Geometry: see drawing. Coordinates: mm, zero at the bounding-box minimum. Round coordinates to 2 decimals unless told otherwise and drop trailing zeros. Loops run counter-clockwise (first coordinate to the right, second up) from the corner with the lowest first, then second, coordinate; pieces in that order, holes last. Notation, with made-up numbers: (81, 79.5) - (136, 79.5) arc R14 ccw to (136, 101.5) - close; hole circle Ø9 at (15.5, -6.5). An arc over 180 degrees is marked (long way). Return JSON: item names as keys, results as strings. Group by question number.
1. Section A-A on y = 260. Return loops of the section in (x, z).
2. First-contact query: pin 1 Ø7.5 at (y, z) = (436.78, 436.78) entering from -X; pin 2 Ø14.5 at (y, z) = (436.78, 82.63) entering from -X; pin 3 Ø5 at (x, z) = (8.5, 111) entering from -Y; pin 4 Ø4 at (x, y) = (7.5, 58) entering from +Z. Flat tips, straight axial feed; report the tip coordinate or a pass-through.
3. Section D-D on x = 10. Return loops of the section in (y, z), and give its area (3 significant figures).
4. Material intervals for probe 1 along Y at (x, z) = (14, 260); probe 2 along Z at (x, y) = (5.5, 171) (1 decimal); probe 3 along Z at (x, y) = (4, 174.5) (1 decimal), sorted ascending.
5. Section C-C on z = 437. Return loops of the section in (x, y).
6. Section B-B on z = 260. Return loops of the section in (x, y), and give its area (3 significant figures).
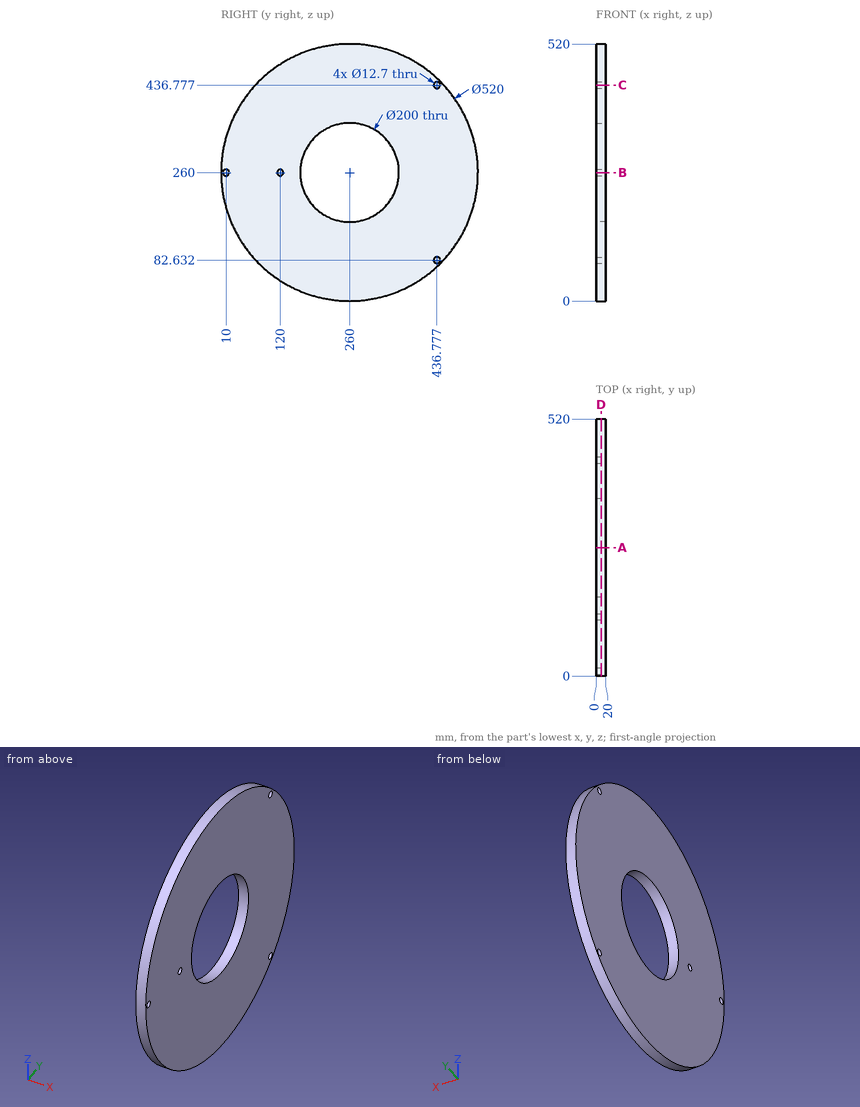
Taken from the geometry:
{
 "1": {"outline": "(0, 0) - (20, 0) - (20, 160) - (0, 160) - close; (0, 360) - (20, 360) - (20, 520) - (0, 520) - close"},
 "2": {"pin 1": "through", "pin 2": "x = 0", "pin 3": "y = 45.2", "pin 4": "z = 426.13"},
 "3": {"outline": "circle Ø520 at (260, 260); hole circle Ø12.7 at (10, 260); hole circle Ø12.7 at (120, 260); hole circle Ø200 at (260, 260); hole circle Ø12.7 at (436.78, 82.63); hole circle Ø12.7 at (436.78, 436.78)", "area": "180,000 mm2"},
 "4": {"probe 1": "0 to 3.65, 16.35 to 113.65, 126.35 to 160, 360 to 520", "probe 2": "15.7 to 214.4, 305.6 to 504.3", "probe 3": "14.5 to 208.1, 311.9 to 505.5"},
 "5": {"outline": "(0, 69.55) - (20, 69.55) - (20, 430.43) - (0, 430.43) - close; (0, 443.12) - (20, 443.12) - (20, 450.45) - (0, 450.45) - close"},
 "6": {"outline": "(0, 0) - (20, 0) - (20, 3.65) - (0, 3.65) - close; (0, 16.35) - (20, 16.35) - (20, 113.65) - (0, 113.65) - close; (0, 126.35) - (20, 126.35) - (20, 160) - (0, 160) - close; (0, 360) - (20, 360) - (20, 520) - (0, 520) - close", "area": "5,890 mm2"}
}
